Model file for the job. Use its own axes, mm. Coordinates: 2 decimals unless noted, no trailing zeros. Order: outer loops, then holes, each group sorted by start corner. A loop starts at its lowest first (then second) coordinate and runs counter-clockwise, first axis right, second up. Notation, with made-up numbers: (66.25, 62.5) -> (78.25, 62.5) arc R11 cw to (78.25, 71.5) -> close; hole circle Ø11 at (-11.75, 29). An arc over 180 degrees is marked (long way). Write item = value, one per line. Start each with the question number.
Q1. Wall check: line 1 (X direction, y = 2.25, z = 92.9); line 2 (X direction, y = 3.5, z = -0.5); line 3 (Z direction, x = -8.5, y = 0.7). Give the ranges that are in metal, low to high. Write a range as from..to.
Q2. Cut at B-B, the plane x = -3. List the corners of the cut face in (y, z).
Q3. Flat gauge pins, fed straight in: pin 1 (1 mm diameter, centred on x = 11.5, y = 1.5, fed in from -Z); pin 2 (1 mm diameter, centred on x = 8.5, y = 0.5, fed in from -Z); pin 3 (1.2 mm diameter, centred on x = -5, y = 1.5, fed in from +Z). Where does each tip first touch, or does it go through?
Q4. Cut at A-A, the plane y = 0.75. Give the number of separate pieces and of enclosed holes in the cut face, plus the area to 3 significant figures.
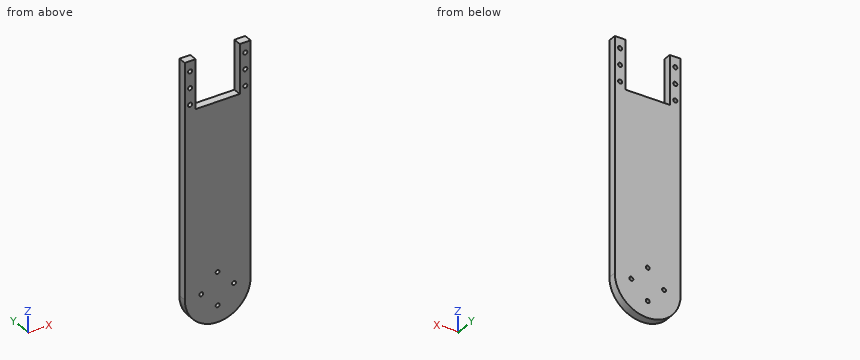
from build123d import *

# Parameters (mm, degrees)
BOSS_EXTRU_1_DEPTH      = 4
ESQUISSE2_R             = 0.955
ESQUISSE2_R_2           = 1
ENL_V_MAT_EXTRU_1_DEPTH = 4
ESQUISSE4_W             = 18
ESQUISSE4_H             = 24
ENL_V_MAT_EXTRU_2_DEPTH = 10
ESQUISSE5_W             = 2.116024011
ESQUISSE5_H             = 24
ESQUISSE5_W_2           = 1.483975989
ENL_V_MAT_EXTRU_3_DEPTH = 10


with BuildPart() as part:
    # Esquisse1 → Boss.-Extru.1 (new body)
    with BuildSketch(Plane(origin=(0, 0, 0), x_dir=(1, 0, 0), z_dir=(0, 1, 0))):
        with BuildLine():
            Line((-16.1, 0), (-16.1, -113.9))
            Line((-16.1, -113.9), (16.1, -113.9))
            Line((16.1, -113.9), (16.1, 0))
            ThreePointArc((16.1, 0), (0, 16.1), (-16.1, 0))
        make_face()
    extrude(amount=BOSS_EXTRU_1_DEPTH)

    # Esquisse2 → Enlèv. mat.-Extru.1 (cut)
    with BuildSketch(Plane(origin=(0, 4, 0), x_dir=(1, 0, 0), z_dir=(0, 1, 0))):
        with Locations(Location((7.975097556, -0.002271435, 0), (0, 0, 270))):
            Circle(ESQUISSE2_R)
        with Locations(Location((-8.024902444, -0.002271435, 0), (0, 0, 270))):
            Circle(ESQUISSE2_R)
        with Locations(Location((-0.024902444, -8.002271435, 0), (0, 0, 270))):
            Circle(ESQUISSE2_R)
        with Locations(Location((-0.024902444, 7.997728565, 0), (0, 0, 270))):
            Circle(ESQUISSE2_R)
        with Locations(Location((-13.5, -108.9, 0), (0, 0, 270))):
            Circle(ESQUISSE2_R_2)
        with Locations(Location((13.5, -108.9, 0), (0, 0, 270))):
            Circle(ESQUISSE2_R_2)
        with Locations(Location((-13.5, -100.9, 0), (0, 0, 270))):
            Circle(ESQUISSE2_R_2)
        with Locations(Location((13.5, -100.9, 0), (0, 0, 270))):
            Circle(ESQUISSE2_R_2)
        with Locations(Location((-13.5, -92.9, 0), (0, 0, 270))):
            Circle(ESQUISSE2_R_2)
        with Locations(Location((13.5, -92.9, 0), (0, 0, 270))):
            Circle(ESQUISSE2_R_2)
    extrude(amount=-ENL_V_MAT_EXTRU_1_DEPTH, mode=Mode.SUBTRACT)

    # Esquisse4 → Enlèv. mat.-Extru.2 (cut)
    with BuildSketch(Plane(origin=(0, 4, 0), x_dir=(1, 0, 0), z_dir=(0, 1, 0))):
        with Locations((0.316024011, -101.9)):
            Rectangle(ESQUISSE4_W, ESQUISSE4_H)
    extrude(amount=-ENL_V_MAT_EXTRU_2_DEPTH, mode=Mode.SUBTRACT)

    # Esquisse5 → Enlèv. mat.-Extru.3 (cut)
    with BuildSketch(Plane(origin=(0, 4, 0), x_dir=(1, 0, 0), z_dir=(0, 1, 0))):
        with Locations((-9.741987995, -101.9)):
            Rectangle(ESQUISSE5_W, ESQUISSE5_H)
        with Locations((10.058012006, -101.9)):
            Rectangle(ESQUISSE5_W_2, ESQUISSE5_H)
    extrude(amount=-ENL_V_MAT_EXTRU_3_DEPTH, mode=Mode.SUBTRACT)


solid = part.part
Here are the results:
q1.line_1 = -16.1..-14.5, -12.5..-10.8, 10.8..12.5, 14.5..16.1
q1.line_2 = -16.09..-8.84, -7.21..7.16, 8.79..16.09
q1.line_3 = -13.67..-0.83, 0.83..89.9
q2.outline = (0, -15.82) -> (4, -15.82) -> (4, 89.9) -> (0, 89.9) -> close
q3.pin_1 = -11.76
q3.pin_2 = -13.97
q3.pin_3 = 89.9
q4.separate_pieces = 1
q4.enclosed_holes = 10
q4.area = 3,530 mm²
